Part model, mm, in its own coordinate system. A direction names the side the tool comes from. Give positions to 0.01 mm unless a question says otherwise; leave off trailing zeros. Order: outer loops, then holes, each group sorted by start corner. A loop starts at its lowest first (then second) coordinate and runs counter-clockwise, first axis right, second up.
from build123d import *

# Parameters (mm, degrees)
SKETCH1_W           = 218
SKETCH1_H           = 30
BOSS_EXTRUDE1_DEPTH = 5
FILLET1_R           = 20
SKETCH2_R           = 10
CUT_EXTRUDE2_DEPTH  = 4
CHAMFER1_SIZE       = 3
SKETCH4_R           = 5
CUT_EXTRUDE3_DEPTH  = 119.159523594
BOSS_EXTRUDE4_DEPTH = 20
SKETCH7_W           = 30
SKETCH7_H           = 21.4
BOSS_EXTRUDE6_DEPTH = 3
SKETCH12_W          = 30.262484152
SKETCH12_H          = 21.4
CUT_EXTRUDE6_DEPTH  = 3
CUT_EXTRUDE7_DEPTH  = 40
CUT_EXTRUDE9_DEPTH  = 40


with BuildPart() as part:
    # Sketch1 → Boss-Extrude1 (new, symmetric)
    with BuildSketch(Plane.XY):
        Rectangle(SKETCH1_W, SKETCH1_H)
    extrude(amount=BOSS_EXTRUDE1_DEPTH, both=True)

    # Fillet1
    fillet1_edges = [part.edges().sort_by_distance(p)[0] for p in [
        (109, -15, 0),
        (-109, -15, 0),
    ]]
    fillet(fillet1_edges, radius=FILLET1_R)

    # Sketch2 → Cut-Extrude2 (cut)
    with BuildSketch(Plane.XY.offset(5)):
        with Locations((-91, 2)):
            Circle(SKETCH2_R)
        with Locations((-31, 2)):
            Circle(SKETCH2_R)
    extrude(amount=-CUT_EXTRUDE2_DEPTH, mode=Mode.SUBTRACT)

    # Chamfer1
    chamfer1_edges = [part.edges().sort_by_distance(p)[0] for p in [
        (-101, 2, 5),
        (-41, 2, 5),
    ]]
    chamfer(chamfer1_edges, length=CHAMFER1_SIZE - 0.0001)  # a hair under: the kernel refuses the full size

    # Sketch3 → Revolve1 (revolve)
    with BuildSketch(Plane(origin=(-61.85, 0, 0), x_dir=(0, 0, -1), z_dir=(1, 0, 0)), mode=Mode.PRIVATE) as revolve1_sk:
        Polygon((-20.856554777, 18.13092454), (-24.491559772, 11.570685315), (8.651987636, -6.794035278), (12.286992632, -0.233796053), align=None)
    revolve(revolve1_sk.sketch.rotate(Axis((-61.85, 11.570685315, 24.491559772), (0, -0.48466733269062345, -0.8746985632905524)), 180), axis=Axis((-61.85, 11.570685315, 24.491559772), (0, -0.48466733269062345, -0.8746985632905524)))

    # Sketch4 → Cut-Extrude3 (cut, through all)
    with BuildSketch(Plane(origin=(0, 13.100880469, 23.643684133), x_dir=(1, 0, 0), z_dir=(0, 0.48466733269062356, 0.8746985632905525))):
        with Locations(Location((-61.85, -1.749397127, 0), (0, 0, 270))):
            Circle(SKETCH4_R)
    extrude(amount=-CUT_EXTRUDE3_DEPTH, mode=Mode.SUBTRACT)

    # Sketch5 → Boss-Extrude4 (add, symmetric)
    with BuildSketch(Plane(origin=(0, 0, 0), x_dir=(0, 0, -1), z_dir=(1, 0, 0))):
        Polygon((5, -15), (-5, -15), (-24.115322554, -63.915136607), (-80.44712563, -74.437688296), (-80.44712563, -84.437688296), (-18.44712563, -75), align=None)
    extrude(amount=BOSS_EXTRUDE4_DEPTH, both=True)

    # Sketch7 → Boss-Extrude6 (add)
    with BuildSketch(Plane(origin=(0, -0.292155586, -0.747611262), x_dir=(1, 0, 0), z_dir=(0, 0.3639801648731982, 0.9314066993418502))):
        with Locations((0, -27.490001314)):
            Rectangle(SKETCH7_W, SKETCH7_H)
    extrude(amount=BOSS_EXTRUDE6_DEPTH)

    # Sketch12 → Cut-Extrude6 (cut)
    with BuildSketch(Plane(origin=(0, -0.292155586, -0.747611262), x_dir=(1, 0, 0), z_dir=(0, 0.3639801648731982, 0.9314066993418502))):
        with Locations((0, -52.608485504)):
            Rectangle(SKETCH12_W, SKETCH12_H)
    extrude(amount=-CUT_EXTRUDE6_DEPTH, mode=Mode.SUBTRACT)

    # Sketch16 → Revolve2 (revolve)
    with BuildSketch(Plane(origin=(0, 0, 0), x_dir=(0, 0, -1), z_dir=(1, 0, 0)), mode=Mode.PRIVATE) as revolve2_sk:
        with BuildLine():
            Line((-52.272833575, -27.565753671), (-52.272833575, -91.206271932))
            Line((-52.272833575, -91.206271932), (-44.772833575, -91.206271932))
            Line((-44.772833575, -91.206271932), (-44.772833575, -81.206271932))
            Line((-44.772833575, -81.206271932), (-47.272833575, -81.206271932))
            Line((-47.272833575, -81.206271932), (-47.272833575, -66.206271932))
            ThreePointArc((-47.272833575, -66.206271932), (-48.101213981, -63.643814293), (-50.272833575, -62.051183895))
            Line((-50.272833575, -62.051183895), (-50.272833575, -39.90745984))
            ThreePointArc((-50.272833575, -39.90745984), (-45.10198049, -32.736606756), (-52.272833575, -27.565753671))
        make_face()
    revolve(revolve2_sk.sketch.rotate(Axis((0, -19.401017973, 52.272833575), (0, -1, 0)), 180), axis=Axis((0, -19.401017973, 52.272833575), (0, -1, 0)))

    # Sketch17 → Cut-Extrude7 (cut)
    with BuildSketch(Plane(origin=(0, 15, 0), x_dir=(1, 0, 0), z_dir=(0, 1, 0))):
        Polygon((-109, 5), (-109, -5), (-105.52, 5), align=None)
    extrude(amount=-CUT_EXTRUDE7_DEPTH, mode=Mode.SUBTRACT)

    # Sketch19 → Cut-Extrude9 (cut)
    with BuildSketch(Plane(origin=(0, 15, 0), x_dir=(1, 0, 0), z_dir=(0, 1, 0))):
        Polygon((109, 5), (105.52, 5), (109, -5), align=None)
    extrude(amount=-CUT_EXTRUDE9_DEPTH, mode=Mode.SUBTRACT)


solid = part.part
Item 1: Which spindle directions (+Z, -Z, +X, -X, +Y, -Y) get a long thin tool onto all of the face, cutting with end or side? Do faces 4 (the face through (-2.253, -86.136, 59.426)), 5 (the face through (-31, 2, 1)), 6 (the face through (-0.22, -80.458, 47.278)). Say none if no direction does.
Item 2: Drill centre lines: probe 1 along Y at (x, z) = (-31, 1.8); probe 2 along Z at (x, y) = (41, 13); probe 3 along Y at (x, z) = (-58, 7.5). Where is each one in solid material? Low to high.
Item 3: Pull direction Y, two halves, no side cores. Call faces 1 (the face through (-63.622, 7.289, 26.864)), 2 (the face through (0, -79, 80.447)), 3 (the face through (-0.21, -50.24, 15.55)): released by +Y, released by -Y, zero draft, split by the parting line, or undercut.
Item 4: Band-saw the part on A-A on x = 12. List the corners of the cut face in (y, z).
Item 5: Drop flat-ended pins along their axis: P1, Ø1.5, axis at x = -9, z = 19, coming from the -Y side; P2, Ø10, axis at x = -92.5, y = 5, coming from the +Z side; P3, Ø11, axis at x = 63, z = 2, coming from the -Y side. Give the stop position or say it passes through.
Item 6: Band-saw the part on D-D on z = 64.5. List the corners of the cut face in (x, y), plus the area to 3 significant figures.
Item 7: Band-saw the part on B-B on x = -59.5. List the corners of the cut face in (y, z).
Working result:
1. face 4: -Y
1. face 5: +Z
1. face 6: none
2. probe 1: y = -15 to -8, 12 to 15
2. probe 2: z = -5 to 5
2. probe 3: y = -5.2 to -1.49, 5.8 to 9.51
3. face 1: released by +Y
3. face 2: zero draft
3. face 3: undercut
4. outline: (-84.44, 80.45) - (-75, 18.45) - (-15, -5) - (15, -5) - (15, 5) - (-15, 5) - (-15.93, 5.36) - (-14.84, 8.16) - (-34.77, 15.95) - (-35.86, 13.15) - (-39.33, 14.51) - (-40.42, 11.71) - (-60.35, 19.5) - (-59.26, 22.3) - (-63.92, 24.12) - (-74.44, 80.45) - close
5. P1: stops at y = -75.2
5. P2: stops at z = 1
5. P3: stops at y = -15
6. outline: (-20, -82.01) - (20, -82.01) - (20, -71.46) - (-20, -71.46) - close
6. area: 422 mm2
7. outline: (-15, -5) - (-12.91, -5) - (-13.02, -5.2) - (-10.65, -6.51) - (7.71, 26.63) - (5.34, 27.94) - (-7.37, 5) - (-15, 5) - close; (-2.93, -10.79) - (-0.56, -12.1) - (3.37, -5) - (15, -5) - (15, 5) - (8.91, 5) - (17.8, 21.04) - (15.43, 22.35) - close
